from build123d import *

# Parameters (mm, degrees)
SKETCH_2_R          = 115
EXTRUDE_2_DEPTH     = 10
EXTRUDE_3_DEPTH     = 5
CUT_EXTRUDE_2_REACH = 164.942
SKETCH_2_6_R        = 4
CUT_EXTRUDE_3_REACH = 164.942
SKETCH_4_R          = 2.1


with BuildPart() as part:
    # Sketch 2 → Extrude 2 (new body)
    with BuildSketch(Plane(origin=(0, 0, 0), x_dir=(1, 0, 0), z_dir=(0, 1, 0))):
        with Locations(Location((0, 0, 0), (0, 0, 270))):
            Circle(SKETCH_2_R)
        Polygon((0, -6.92820323), (6, -3.464101615), (6, 3.464101615), (0, 6.92820323), (-6, 3.464101615), (-6, -3.464101615), align=None, mode=Mode.SUBTRACT)
    extrude(amount=EXTRUDE_2_DEPTH)

    # Sketch 2_4 → Extrude 3 (add)
    with BuildSketch(Plane(origin=(0, 0, 0), x_dir=(1, 0, 0), z_dir=(0, 1, 0))):
        Polygon((0, -6.92820323), (6, -3.464101615), (6, 3.464101615), (0, 6.92820323), (-6, 3.464101615), (-6, -3.464101615), align=None)
    extrude(amount=EXTRUDE_3_DEPTH)

    # Sketch 2_6 → Cut-Extrude 2 (cut, up to next)
    with BuildSketch(Plane(origin=(0, 0, 0), x_dir=(1, 0, 0), z_dir=(0, 1, 0)), mode=Mode.PRIVATE) as cut_extrude_2_sk1:
        with Locations(Location((0, 0, 0), (0, 0, 270))):
            Circle(SKETCH_2_6_R)
    cut_extrude_2_tool1 = extrude(cut_extrude_2_sk1.sketch, amount=CUT_EXTRUDE_2_REACH, mode=Mode.PRIVATE) & part.part
    add(cut_extrude_2_tool1.solids().sort_by_distance((0, 0, 0))[0], mode=Mode.SUBTRACT)

    # Sketch 4 → Cut-Extrude 3 (cut, up to next)
    with BuildSketch(Plane(origin=(0, 10, 0), x_dir=(1, 0, 0), z_dir=(0, 1, 0)), mode=Mode.PRIVATE) as cut_extrude_3_sk1:
        with Locations(Location((-50, -86.602540378, 0), (0, 0, 270))):
            Circle(SKETCH_4_R)
    cut_extrude_3_tool1 = extrude(cut_extrude_3_sk1.sketch, amount=-CUT_EXTRUDE_3_REACH, mode=Mode.PRIVATE) & part.part
    # Sketch 4 → Cut-Extrude 3 (cut, up to next)
    with BuildSketch(Plane(origin=(0, 10, 0), x_dir=(1, 0, 0), z_dir=(0, 1, 0)), mode=Mode.PRIVATE) as cut_extrude_3_sk2:
        with Locations(Location((50, -86.602540378, 0), (0, 0, 270))):
            Circle(SKETCH_4_R)
    cut_extrude_3_tool2 = extrude(cut_extrude_3_sk2.sketch, amount=-CUT_EXTRUDE_3_REACH, mode=Mode.PRIVATE) & part.part
    add(cut_extrude_3_tool1.solids().sort_by_distance((-50, 10, 86.60254))[0], mode=Mode.SUBTRACT)
    add(cut_extrude_3_tool2.solids().sort_by_distance((50, 10, 86.60254))[0], mode=Mode.SUBTRACT)


solid = part.part
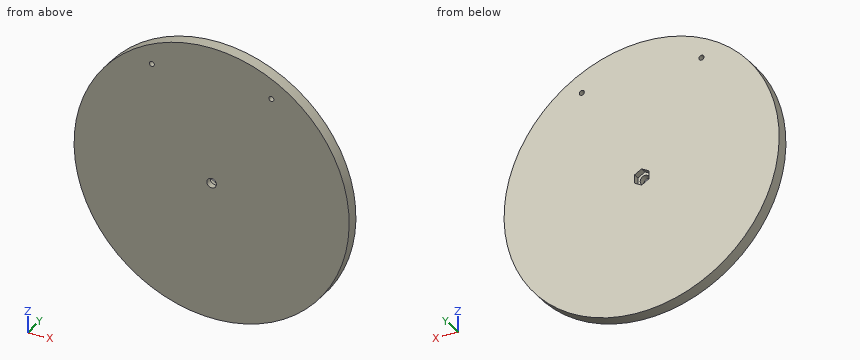
Input: part model. Units: mm. Frame: model coordinates. Give positions to 0.01 mm unless a question says otherwise; leave off trailing zeros. Write each loop counter-clockwise with the first axis right and the second up, starting at its lowest first coordinate (ties: lowest second). Pieces come first, ordered by that corner, then holes. Notation, with made-up numbers: (27.25, 15) -> (70.25, 15) arc R25 cw to (70.25, 38) -> close; hole circle Ø10 at (63.5, 24.25). An arc over 180 degrees is marked (long way). Use one line per item in the form item = value. Start each with the question number.
1) Pin query (flat end, axial travel): pin 1 (6 mm diameter, centred on x = -2, z = -0.5, fed in from +Y); pin 2 (1 mm diameter, centred on x = 1, y = 8, fed in from -Z); pin 3 (3.5 mm diameter, centred on x = 50, z = 86.6, fed in from -Y) (3 decimals); pin 4 (3 mm diameter, centred on y = 6, z = -76.5, fed in from +X). Return the tip coordinate at first contact, or that it passes through.
2) Section query A-A on y = 8. Return the cut outline in (x, z).
3) Section query C-C on z = -24. Return the cut outline in (x, y), then the cut area to 3 significant figures.
4) Ray query, probe 1 along X at (y, z) = (1.1, 0); probe 2 along X at (y, z) = (2.5, 1); probe 3 along X at (y, z) = (7.5, 22.5). Return the intervals inside material, ascending. Write a range as from..to.
5) Section query B-B on x = 91.5. Return the cut outline in (y, z).
Outcome:
q1.pin_1 = 5
q1.pin_2 = -115
q1.pin_3 = through
q1.pin_4 = 87.18
q2.outline = circle Ø230 at (0, 0); hole circle Ø4.2 at (-50, 86.6); hole (-6, -3.46) -> (0, -6.93) -> (6, -3.46) -> (6, 3.46) -> (0, 6.93) -> (-6, 3.46) -> close; hole circle Ø4.2 at (50, 86.6)
q3.outline = (-112.47, 0) -> (112.47, 0) -> (112.47, 10) -> (-112.47, 10) -> close
q3.area = 2,250 mm^2
q4.probe_1 = -115..-4, 4..115
q4.probe_2 = -115..-3.87, 3.87..115
q4.probe_3 = -112.78..112.78
q5.outline = (0, -69.66) -> (10, -69.66) -> (10, 69.66) -> (0, 69.66) -> close
